```python
from build123d import *

# Parameters (mm, degrees)
SKETCH1_R           = 15
BOSS_EXTRUDE1_DEPTH = 15
CUT_EXTRUDE1_DEPTH  = 15


with BuildPart() as part:
    # Sketch1 → Boss-Extrude1 (new body)
    with BuildSketch(Plane(origin=(0, 0, 0), x_dir=(1, 0, 0), z_dir=(0, 1, 0))):
        with Locations(Location((0, 0, 0), (0, 0, 270))):
            Circle(SKETCH1_R)
    extrude(amount=BOSS_EXTRUDE1_DEPTH)

    # Sketch2 → Cut-Extrude1 (cut)
    with BuildSketch(Plane(origin=(0, 15, 0), x_dir=(1, 0, 0), z_dir=(0, 1, 0))):
        with BuildLine():
            Line((-0.78062475, 12.269997998), (-3.69895875, 8.625))
            ThreePointArc((-3.69895875, 8.625), (-3.819721819, 7.566987298), (-2.918334001, 7))
            Line((-2.918334001, 7), (2.918334001, 7))
            ThreePointArc((2.918334001, 7), (3.819721819, 7.566987298), (3.69895875, 8.625))
            Line((3.69895875, 8.625), (0.78062475, 12.269997998))
            ThreePointArc((0.78062475, 12.269997998), (0, 12.644997998), (-0.78062475, 12.269997998))
        make_face()
        with BuildLine():
            Line((8.625, -3.69895875), (12.269997998, -0.78062475))
            ThreePointArc((12.269997998, -0.78062475), (12.644997998, 0), (12.269997998, 0.78062475))
            Line((12.269997998, 0.78062475), (8.625, 3.69895875))
            ThreePointArc((8.625, 3.69895875), (7.566987298, 3.819721819), (7, 2.918334001))
            Line((7, 2.918334001), (7, -2.918334001))
            ThreePointArc((7, -2.918334001), (7.566987298, -3.819721819), (8.625, -3.69895875))
        make_face()
        with BuildLine():
            Line((-3, -4), (3, -4))
            ThreePointArc((3, -4), (3.707106781, -3.707106781), (4, -3))
            Line((4, -3), (4, 3))
            ThreePointArc((4, 3), (3.707106781, 3.707106781), (3, 4))
            Line((3, 4), (-3, 4))
            ThreePointArc((-3, 4), (-3.707106781, 3.707106781), (-4, 3))
            Line((-4, 3), (-4, -3))
            ThreePointArc((-4, -3), (-3.707106781, -3.707106781), (-3, -4))
        make_face()
        with BuildLine():
            Line((-8.625, 3.69895875), (-12.269997998, 0.78062475))
            ThreePointArc((-12.269997998, 0.78062475), (-12.644997998, 0), (-12.269997998, -0.78062475))
            Line((-12.269997998, -0.78062475), (-8.625, -3.69895875))
            ThreePointArc((-8.625, -3.69895875), (-7.566987298, -3.819721819), (-7, -2.918334001))
            Line((-7, -2.918334001), (-7, 2.918334001))
            ThreePointArc((-7, 2.918334001), (-7.566987298, 3.819721819), (-8.625, 3.69895875))
        make_face()
    extrude(amount=-CUT_EXTRUDE1_DEPTH, mode=Mode.SUBTRACT)


solid = part.part
```
Can you work these out from the model? Positions are in its coordinate system, mm. A direction names the side the tool comes from. Coordinates: 2 decimals unless noted, no trailing zeros. Loops run counter-clockwise (first coordinate to the right, second up) from the corner with the lowest first, then second, coordinate; pieces in that order, holes last.
Item 1: Please list where these lines run through material, in increasing order: L1, parallel to X at y = 9.25, z = -3.5; L2, parallel to X at y = 7.75, z = 2; L3, parallel to Z at x = -1.25, y = 13.
Answers below:
L1: x = -14.59 to -8.87, -7.19 to -3.87, 3.87 to 7.19, 8.87 to 14.59
L2: x = -14.87 to -10.75, -7 to -4, 4 to 7, 10.75 to 14.87
L3: z = -14.95 to -11.68, -7 to -4, 4 to 14.95
Item 2: Which directions (+Z, -Z, +X, -X, +Y, -Y) give clear straight access to the entire face, cutting with the end or side of a thin tool? Please do faces 4 (the face through (0, 0, 6)), 5 (the face through (-7, 8, 0)).
Answers below:
face 4: +Z, -Z, +X, -X, -Y
face 5: +Y, -Y
Item 3: Suppose I cut it at C-C (y = 12). Please give me the cut outline in (x, z) (3 decimals).
Answers below:
outline: circle Ø30 at (0, 0); hole (-12.27, -0.781) - (-8.625, -3.699) arc R1 ccw to (-7, -2.918) - (-7, 2.918) arc R1 ccw to (-8.625, 3.699) - (-12.27, 0.781) arc R1 ccw to start; hole (-4, -3) arc R1 ccw to (-3, -4) - (3, -4) arc R1 ccw to (4, -3) - (4, 3) arc R1 ccw to (3, 4) - (-3, 4) arc R1 ccw to (-4, 3) - close; hole (-3.699, -8.625) - (-0.781, -12.27) arc R1 ccw to (0.781, -12.27) - (3.699, -8.625) arc R1 ccw to (2.918, -7) - (-2.918, -7) arc R1 ccw to start; hole (7, -2.918) arc R1 ccw to (8.625, -3.699) - (12.27, -0.781) arc R1 ccw to (12.27, 0.781) - (8.625, 3.699) arc R1 ccw to (7, 2.918) - close
Item 4: Suppose I cut it at A-A (z = 0). Please give me the cut outline in (x, y) (3 decimals).
Answers below:
outline: (-15, 0) - (-12.645, 0) - (-12.645, 15) - (-15, 15) - close; (-7, 0) - (-4, 0) - (-4, 15) - (-7, 15) - close; (4, 0) - (7, 0) - (7, 15) - (4, 15) - close; (12.645, 0) - (15, 0) - (15, 15) - (12.645, 15) - close
Item 5: Suppose I cut it at D-D (x = 10.75). Please give me the cut outline in (y, z), then the cut area to 3 significant figures.
Answers below:
outline: (0, -10.46) - (15, -10.46) - (15, -2) - (0, -2) - close; (0, 2) - (15, 2) - (15, 10.46) - (0, 10.46) - close
area: 254 mm2
Item 6: If we mould it in two halves opening along Z, with no side actions, what happens to faces 1 (the face through (0, 15, 6)), 2 (the face through (0.66, 7.395, -14.985)), 3 (the face through (0.013, 7.605, -12.645))? For each: released by +Z, released by -Z, zero draft, split by the parting line, or undercut.
Answers below:
face 1: zero draft
face 2: split by the parting line
face 3: undercut
Item 7: I'm going to push flat-ended pins straight in: pin 1 (4 mm diameter, centred on x = -8.5, y = 3.5, fed in from -Z); pin 2 (8 mm diameter, centred on y = 2, z = -9.5, fed in from -X); pin 3 (3 mm diameter, centred on x = -11.5, y = 10.5, fed in from +Z); pin 4 (4 mm diameter, centred on x = -6.5, z = 8.5, fed in from -Y). Where does each tip first touch, or does it pass through?
Answers below:
pin 1: stops at z = -13.52
pin 2: stops at x = -13.96
pin 3: stops at z = 11.18
pin 4: stops at y = 0
Item 8: Suppose I cut it at B-B (x = 0). Please give me the cut outline in (y, z) (3 decimals), then the cut area to 3 significant figures.
Answers below:
outline: (0, -15) - (15, -15) - (15, -12.645) - (0, -12.645) - close; (0, -7) - (15, -7) - (15, -4) - (0, -4) - close; (0, 4) - (15, 4) - (15, 15) - (0, 15) - close
area: 245 mm2
